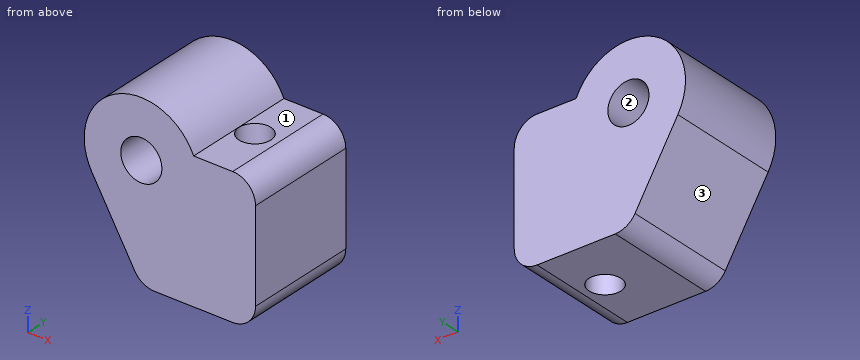
from build123d import *

# Parameters (mm, degrees)
SKETCH1_R           = 2.286
BOSS_EXTRUDE1_DEPTH = 12.7
SKETCH2_R           = 1.778
CUT_EXTRUDE1_DEPTH  = 24.554990979
FILLET1_R           = 2.54


with BuildPart() as part:
    # Sketch1 → Boss-Extrude1 (new body)
    with BuildSketch(Plane(origin=(0, 0, 0), x_dir=(1, 0, 0), z_dir=(0, 1, 0))):
        with BuildLine():
            Line((-5.499261314, 3.175), (0, 12.7))
            Line((0, 12.7), (12.7, 12.7))
            Line((12.7, 12.7), (12.7, -2.54))
            Line((12.7, -2.54), (5.819871133, -2.54))
            ThreePointArc((5.819871133, -2.54), (-2.861992997, -5.668465056), (-5.499261314, 3.175))
        make_face()
        with Locations(Location((0, 0, 0), (0, 0, 270))):
            Circle(SKETCH1_R, mode=Mode.SUBTRACT)
    extrude(amount=BOSS_EXTRUDE1_DEPTH)

    # Sketch2 → Cut-Extrude1 (cut, through all)
    with BuildSketch(Plane.XY.offset(2.54)):
        with Locations((7.62, 6.35)):
            Circle(SKETCH2_R)
    extrude(amount=-CUT_EXTRUDE1_DEPTH, mode=Mode.SUBTRACT)

    # Fillet1
    fillet1_edges = [part.edges().sort_by_distance(p)[0] for p in [
        (0, 6.35, -12.7),
        (12.7, 6.35, -12.7),
        (12.7, 6.35, 2.54),
    ]]
    fillet(fillet1_edges, radius=FILLET1_R)


solid = part.part
Here's how the part is built. I have some questions about the finished solid (model axes, mm). Face numbers are marked on the shaded views. Round coordinates to 2 decimals unless told otherwise and drop trailing zeros. Order: outer loops, then holes, each group sorted by start corner. A loop starts at its lowest first (then second) coordinate and runs counter-clockwise, first axis right, second up. Notation, with made-up numbers: M -18,-7 L 12,-7 A24 ccw 12,18 Z; hole C -35,44 d6. An arc over 180 degrees is marked long. One line per question, with ' | ' between items.
1) Imagine slicing it at B-B, the plane x = -2. Write out the boundary of the cut face in (y, z).
Checked values:
outline: M 0,-9.24 L 12.7,-9.24 L 12.7,-1.11 L 0,-1.11 Z; M 0,1.11 L 12.7,1.11 L 12.7,6.03 L 0,6.03 Z
2) Imagine slicing it at A-A, the plane y = 6.35. Write out the boundary of the cut face in (x, z) (3 decimals), plus the area to 3 significant figures.
Checked values:
outline: M -5.499,-3.175 L -0.733,-11.43 A2.54 ccw 1.466,-12.7 L 5.842,-12.7 L 5.842,2.54 L 5.82,2.54 A6.35 ccw long Z; M 9.398,-12.7 L 10.16,-12.7 A2.54 ccw 12.7,-10.16 L 12.7,0 A2.54 ccw 10.16,2.54 L 9.398,2.54 Z; hole C 0,0 d4.572 | area: 213 mm²
3) I'm going to push flat-ended pins straight in: pin 1 Ø2 at (x, y) = (-2, 8.5) entering from +Z; pin 2 Ø4 at (x, y) = (-1.5, 7.5) entering from -Z; pin 3 Ø3.5 at (x, y) = (8, 9) entering from +Z. Where does each tip first touch, or does it pass through?
Checked values:
pin 1: stops at z = 6.27 | pin 2: stops at z = -12.51 | pin 3: stops at z = 2.54
4) We'd pull the mould along X, two halves only. Please class the marked faces 1, 2 and 3: released by +X, released by -X, zero draft, split by the parting line, or undercut.
Checked values:
face 1: zero draft | face 2: undercut | face 3: released by -X
5) Imagine slicing it at C-C, the plane z = 1.5. Write out the boundary of the cut face in (x, y), plus the area to 3 significant figures.
Checked values:
outline: M -6.17,0 L -1.73,0 L -1.73,12.7 L -6.17,12.7 Z; M 1.73,0 L 12.21,0 L 12.21,12.7 L 1.73,12.7 Z; hole C 7.62,6.35 d3.56 | area: 180 mm²
6) Imagine slicing it at D-D, the plane y = 9.25. Write out the boundary of the cut face in (x, z) (3 decimals).
Checked values:
outline: M -5.499,-3.175 L -0.733,-11.43 A2.54 ccw 1.466,-12.7 L 10.16,-12.7 A2.54 ccw 12.7,-10.16 L 12.7,0 A2.54 ccw 10.16,2.54 L 5.82,2.54 A6.35 ccw long Z; hole C 0,0 d4.572
7) I need wall thicknesses on line 1 (Z direction, x = -0.5, y = 1.75); line 2 (X direction, y = 10.25, z = 2); line 3 (Z direction, x = -2, y = 1). Which ranges of each line are inside material? Lowest first, please.
Checked values:
line 1: z = -11.77 to -2.23, 2.23 to 6.33 | line 2: x = -6.03 to -1.11, 1.11 to 11.73 | line 3: z = -9.24 to -1.11, 1.11 to 6.03
